from build123d import *

# Parameters (mm, degrees)
SKETCH1_R           = 2.5
BOSS_EXTRUDE1_DEPTH = 160
FILLET1_R           = 1.47
SKETCH2_R           = 1.5
CUT_EXTRUDE1_DEPTH  = 161.913672508


with BuildPart() as part:
    # Sketch1 → Boss-Extrude1 (new body)
    with BuildSketch(Plane.XY):
        Polygon((2.860553032, 3.9), (6, 7.039446968), (6, 8.2), (3.1, 8.2), (3.1, 10), (10, 10), (10, 3.1), (8.2, 3.1), (8.2, 6), (7.039446968, 6), (3.9, 2.860553032), (3.9, 0), (3.9, -2.860553032), (7.039446968, -6), (8.2, -6), (8.2, -3.1), (10, -3.1), (10, -10), (3.1, -10), (3.1, -8.2), (6, -8.2), (6, -7.039446968), (2.860553032, -3.9), (0, -3.9), (-2.860553032, -3.9), (-6, -7.039446968), (-6, -8.2), (-3.1, -8.2), (-3.1, -10), (-10, -10), (-10, -3.1), (-8.2, -3.1), (-8.2, -6), (-7.039446968, -6), (-3.9, -2.860553032), (-3.9, 0), (-3.9, 2.860553032), (-7.039446968, 6), (-8.2, 6), (-8.2, 3.1), (-10, 3.1), (-10, 10), (-3.1, 10), (-3.1, 8.2), (-6, 8.2), (-6, 7.039446968), (-2.860553032, 3.9), (0, 3.9), align=None)
        Circle(SKETCH1_R, mode=Mode.SUBTRACT)
    extrude(amount=BOSS_EXTRUDE1_DEPTH)

    # Fillet1
    fillet1_edges = [part.edges().sort_by_distance(p)[0] for p in [
        (10, -10, 80),
        (-10, -10, 80),
        (-10, 10, 80),
        (10, 10, 80),
    ]]
    fillet(fillet1_edges, radius=FILLET1_R)

    # Sketch2 → Cut-Extrude1 (cut, through all)
    with BuildSketch(Plane(origin=(3.9, 0, 0), x_dir=(0, 0, -1), z_dir=(1, 0, 0))):
        with Locations(Location((-150, 0, 0), (0, 0, 90))):
            Circle(SKETCH2_R)
        with Locations(Location((-79.29, 0, 0), (0, 0, 90))):
            Circle(SKETCH2_R)
        with Locations(Location((-10, 0, 0), (0, 0, 90))):
            Circle(SKETCH2_R)
    extrude(amount=-CUT_EXTRUDE1_DEPTH, mode=Mode.SUBTRACT)


solid = part.part
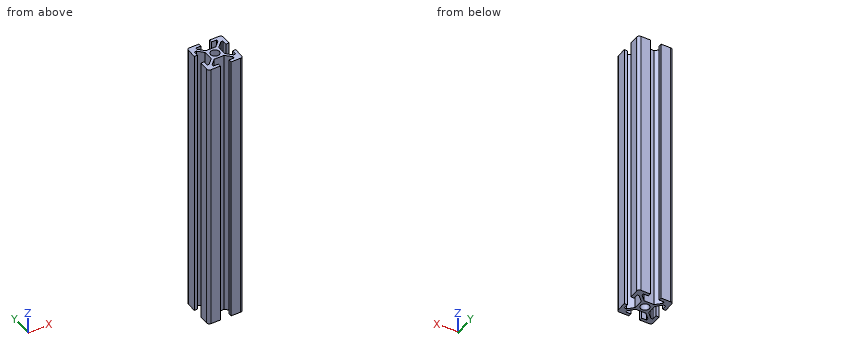
Work out the finished part from the listing and answer in its coordinate system (mm). Round coordinates to 2 decimals unless told otherwise and drop trailing zeros. Order: outer loops, then holes, each group sorted by start corner. A loop starts at its lowest first (then second) coordinate and runs counter-clockwise, first axis right, second up. Notation, with made-up numbers: M 70.25,-12 L 124.25,-12 A22 cw 124.25,-5 Z; hole C 43,44 d1. An arc over 180 degrees is marked long. Put each result on its own line as item: value. Start each with the question number.
Q1. Flat-ended cylindrical pins translate along their axes: pin 1 (6 mm diameter, centred on x = 0, z = 28.5, fed in from -Y); pin 2 (2 mm diameter, centred on x = 1, z = 33, fed in from -Y); pin 3 (1.8 mm diameter, centred on y = 0, z = 150, fed in from +X); pin 4 (3 mm diameter, centred on y = 1, z = 93, fed in from -X). Find the tip coordinate at first contact, or state that the pin passes through.
Q2. Straight lines are drawn through the part: L1, parallel to Z at x = -3.1, y = 0; L2, parallel to Y at x = -8.25, z = 114; L3, parallel to Y at x = -2.8, z = 10. For each, find the intervals that lie inside material, in ascending order. Write a range as [from, to].
Q3. Section B-B, the plane x = 0 is taken. Write down the section's boundary in (y, z), and give its area (3 significant figures).
Q4. Section A-A, the plane y = 0 is taken. Give the number of separate pieces and of enclosed holes in the cut face, and give its area (3 significant figures).
Findings below:
1. pin 1: stops at y = -4.04
1. pin 2: stops at y = -3.9
1. pin 3: passes through
1. pin 4: stops at x = -3.9
2. L1: z = [0, 8.5], [11.5, 77.79], [80.79, 148.5], [151.5, 160]
2. L2: y = [-10, -3.1], [3.1, 10]
2. L3: y = [-3.9, -1.5], [1.5, 3.9]
3. outline: M -3.9,0 L -2.5,0 L -2.5,160 L -3.9,160 Z; M 2.5,0 L 3.9,0 L 3.9,160 L 2.5,160 Z
3. area: 448 mm^2
4. separate pieces: 8
4. enclosed holes: 0
4. area: 423 mm^2
